CAD build for the part. Positions are in the model's coordinates, mm. A direction names the side the tool comes from. Coordinates: 2 decimals unless noted, no trailing zeros. Order: outer loops, then holes, each group sorted by start corner. A loop starts at its lowest first (then second) coordinate and runs counter-clockwise, first axis right, second up. Notation, with made-up numbers: (30, 23.25) - (84, 23.25) arc R28 ccw to (84, 53.25) - close; hole circle Ø9 at (82, 64). An arc over 180 degrees is marked (long way). Use one line per item in the form item = value.
```python
from build123d import *

# Parameters (mm, degrees)
SKETCH1_R                 = 14
BOSS_EXTRUDE1_DEPTH       = 18.5
CUT_EXTRUDE1_START        = -13.5
SKETCH2_R                 = 14
SKETCH2_R_2               = 5
CUT_EXTRUDE1_DEPTH        = 13.5
SKETCH3_R                 = 4
CUT_EXTRUDE2_DEPTH        = 22.5
CUT_EXTRUDE3_DEPTH        = 3.75
SKETCH8_R                 = 12.271364757
SKETCH8_R_2               = 6.141449245
CUT_EXTRUDE4_DEPTH        = 2.75
CIRPATTERN1_COUNT         = 4
SKETCH11_R                = 1.5
CUT_EXTRUDE5_DEPTH        = 3
SKETCH12_R                = 21.13637798
CUT_EXTRUDE6_DEPTH        = 17
BOSS_EXTRUDE2_START       = -1.5
BOSS_EXTRUDE2_OUTLINE_R   = 1.5
BOSS_EXTRUDE2_OUTLINE_R_2 = 1.517060808
BOSS_EXTRUDE2_OUTLINE_R_3 = 4
BOSS_EXTRUDE2_OUTLINE_R_4 = 1.426709917
BOSS_EXTRUDE2_DEPTH       = 1.5
FILLET1_R                 = 2.5
SKETCH14_R                = 1.5
SKETCH14_R_2              = 5
CUT_EXTRUDE7_DEPTH        = 14.5


# Read off the part's stored shape, not the designer's step: Boss-Extrude2
with BuildPart() as part:
    # Sketch1 → Boss-Extrude1 (new body)
    with BuildSketch(Plane.XY):
        Circle(SKETCH1_R)
    extrude(amount=BOSS_EXTRUDE1_DEPTH)

    # Sketch2 → Cut-Extrude1 (cut)
    with BuildSketch(Plane.XY.offset(18.5).offset(CUT_EXTRUDE1_START)):
        Circle(SKETCH2_R)
        Circle(SKETCH2_R_2, mode=Mode.SUBTRACT)
    extrude(amount=CUT_EXTRUDE1_DEPTH, mode=Mode.SUBTRACT)

    # Sketch3 → Cut-Extrude2 (cut)
    with BuildSketch(Plane.XY.offset(18.5)):
        Circle(SKETCH3_R)
    extrude(amount=-CUT_EXTRUDE2_DEPTH, mode=Mode.SUBTRACT)

    # Sketch6 → Cut-Revolve1 (revolve, cut)
    with BuildSketch(Plane(origin=(0, 0, 0), x_dir=(0, 0, -1), z_dir=(1, 0, 0)), mode=Mode.PRIVATE) as cut_revolve1_sk:
        Polygon((-4.949121361, 14), (3.777639186, 16.199586118), (5.061522468, 10.233304984), align=None)
    revolve(cut_revolve1_sk.sketch.rotate(Axis((0, 0, 19.921792725), (0, 0, -1)), 90), axis=Axis((0, 0, 19.921792725), (0, 0, -1)), mode=Mode.SUBTRACT)

    # Sketch7 → Cut-Extrude3 (cut)
    with BuildSketch(Plane(origin=(0, 0, 0), x_dir=(-1, 0, 0), z_dir=(0, 0, -1))):
        with BuildLine():
            Line((3, 15.639460569), (3, 11.87697352))
            add(Edge.make_bspline(
                [(3, 11.87697352), (3.121054504, 3.206614769), (11.87697352, 3)],
                knots=[0, 0, 0, 1, 1, 1], degree=2))
            Line((11.87697352, 3), (17.86108213, 3))
            Line((17.86108213, 3), (14.869027825, 14.316513241))
            Line((14.869027825, 14.316513241), (3, 15.639460569))
        make_face()
    cut_extrude3 = extrude(amount=-CUT_EXTRUDE3_DEPTH, mode=Mode.SUBTRACT)

    # Sketch8 → Cut-Extrude4 (cut)
    with BuildSketch(Plane.XY.offset(5)):
        Circle(SKETCH8_R)
        Circle(SKETCH8_R_2, mode=Mode.SUBTRACT)
    extrude(amount=-CUT_EXTRUDE4_DEPTH, mode=Mode.SUBTRACT)

    # Sketch9 → Cut-Revolve2 (revolve, cut)
    with BuildSketch(Plane(origin=(0, 0, 0), x_dir=(1, 0, 0), z_dir=(0, 1, 0)), mode=Mode.PRIVATE) as cut_revolve2_sk:
        Polygon((-12.001476603, -2.22152714), (-13.001507243, -5.36905248), (-11.155114973, -5.36905248), align=None)
    revolve(cut_revolve2_sk.sketch.rotate(Axis((0, 0, -1.742471472), (0, 0, 1)), 180), axis=Axis((0, 0, -1.742471472), (0, 0, 1)), mode=Mode.SUBTRACT)

    # Sketch10 → Cut-Revolve3 (revolve, cut)
    with BuildSketch(Plane(origin=(0, 0, 0), x_dir=(1, 0, 0), z_dir=(0, 1, 0)), mode=Mode.PRIVATE) as cut_revolve3_sk:
        Polygon((-5, -5), (-6.141449245, -2.28305418), (-6.572257958, -5.413209842), align=None)
    revolve(cut_revolve3_sk.sketch.rotate(Axis((0, 0, 0), (0, 0, -1)), 180), axis=Axis((0, 0, 0), (0, 0, -1)), mode=Mode.SUBTRACT)

    # CirPattern1: Cut-Extrude3 ×4 about axis
    cirpattern1_axis = Axis((0, 0, 3.75), (0, 0, 1))
    for i in range(1, CIRPATTERN1_COUNT):
        add(cut_extrude3.rotate(cirpattern1_axis, i * 360 / CIRPATTERN1_COUNT), mode=Mode.SUBTRACT)

    # Sketch11 → Cut-Extrude5 (cut)
    with BuildSketch(Plane(origin=(0, 0, 0), x_dir=(-1, 0, 0), z_dir=(0, 0, -1))):
        with Locations((0, 8)):
            Circle(SKETCH11_R)
        with Locations((0, -8)):
            Circle(SKETCH11_R)
        with Locations((-10, 0)):
            Circle(SKETCH11_R)
        with Locations((10, 0)):
            Circle(SKETCH11_R)
    extrude(amount=-CUT_EXTRUDE5_DEPTH, mode=Mode.SUBTRACT)

    # Sketch12 → Cut-Extrude6 (cut)
    with BuildSketch(Plane.XY.offset(18.5)):
        Circle(SKETCH12_R)
    extrude(amount=-CUT_EXTRUDE6_DEPTH, mode=Mode.SUBTRACT)

    # Boss-Extrude2 outline → Boss-Extrude2 (add)
    # profile 1 of 7: a face of its own
    with BuildSketch(Plane(origin=(0, 0, 0), x_dir=(-1, 0, 0), z_dir=(0, 0, -1)).offset(BOSS_EXTRUDE2_START)):
        with BuildLine():
            add(Edge.make_bspline(
                [(3.00190242, 11.760729011), (3.000755095, 11.818659857), (3, 11.87697352)],
                knots=[0.993159083, 0.993159083, 0.993159083, 1, 1, 1], degree=2))
            Line((3, 11.87697352), (3, 19.773719933))
            ThreePointArc((3, 19.773719933), (-0.004378174, 19.999999521), (-3.00865699, 19.772404586))
            Line((-3.00865699, 19.772404586), (-3.008656992, 11.602060374))
            add(Edge.make_bspline(
                [(-5.368896851, 5.233886038), (-3.175302873, 7.384008673), (-3.008656992, 11.602060374)],
                knots=[0.4948048, 0.4948048, 0.4948048, 0.984177857, 0.984177857, 0.984177857], degree=2))
            add(Edge.make_bspline(
                [(-5.368896851, 5.233886038), (-7.55686142, 3.085160323), (-11.760729011, 3.00190242)],
                knots=[0.496734279, 0.496734279, 0.496734279, 0.993159083, 0.993159083, 0.993159083], degree=2))
            add(Edge.make_bspline(
                [(-11.760729011, 3.00190242), (-11.818659857, 3.000755095), (-11.87697352, 3)],
                knots=[0.993159083, 0.993159083, 0.993159083, 1, 1, 1], degree=2))
            Line((-11.87697352, 3), (-19.773719933, 3))
            ThreePointArc((-19.773719933, 3), (-19.999999521, -0.004378174), (-19.772404586, -3.00865699))
            Line((-19.772404586, -3.00865699), (-11.602060374, -3.008656992))
            add(Edge.make_bspline(
                [(-5.233886038, -5.368896851), (-7.384008673, -3.175302873), (-11.602060374, -3.008656992)],
                knots=[0.4948048, 0.4948048, 0.4948048, 0.984177857, 0.984177857, 0.984177857], degree=2))
            add(Edge.make_bspline(
                [(-5.233886038, -5.368896851), (-3.085160323, -7.55686142), (-3.00190242, -11.760729011)],
                knots=[0.496734279, 0.496734279, 0.496734279, 0.993159083, 0.993159083, 0.993159083], degree=2))
            add(Edge.make_bspline(
                [(-3.00190242, -11.760729011), (-3.000755095, -11.818659857), (-3, -11.87697352)],
                knots=[0.993159083, 0.993159083, 0.993159083, 1, 1, 1], degree=2))
            Line((-3, -11.87697352), (-3, -19.773719933))
            ThreePointArc((-3, -19.773719933), (0.004378174, -19.999999521), (3.00865699, -19.772404586))
            Line((3.00865699, -19.772404586), (3.008656992, -11.602060374))
            add(Edge.make_bspline(
                [(5.368896851, -5.233886038), (3.175302873, -7.384008673), (3.008656992, -11.602060374)],
                knots=[0.4948048, 0.4948048, 0.4948048, 0.984177857, 0.984177857, 0.984177857], degree=2))
            add(Edge.make_bspline(
                [(5.368896851, -5.233886038), (7.55686142, -3.085160323), (11.760729011, -3.00190242)],
                knots=[0.496734279, 0.496734279, 0.496734279, 0.993159083, 0.993159083, 0.993159083], degree=2))
            add(Edge.make_bspline(
                [(11.760729011, -3.00190242), (11.818659857, -3.000755095), (11.87697352, -3)],
                knots=[0.993159083, 0.993159083, 0.993159083, 1, 1, 1], degree=2))
            Line((11.87697352, -3), (19.773719933, -3))
            ThreePointArc((19.773719933, -3), (19.999999521, 0.004378174), (19.772404586, 3.00865699))
            Line((19.772404586, 3.00865699), (11.602060374, 3.008656992))
            add(Edge.make_bspline(
                [(5.233886023, 5.368896867), (7.384008658, 3.175302874), (11.602060374, 3.008656992)],
                knots=[0.494804799, 0.494804799, 0.494804799, 0.984177857, 0.984177857, 0.984177857], degree=2))
            add(Edge.make_bspline(
                [(5.233886023, 5.368896867), (3.085160322, 7.556861435), (3.00190242, 11.760729011)],
                knots=[0.496734281, 0.496734281, 0.496734281, 0.993159083, 0.993159083, 0.993159083], degree=2))
        make_face()
        with Locations((0, -8)):
            Circle(BOSS_EXTRUDE2_OUTLINE_R, mode=Mode.SUBTRACT)
        with Locations((-10, 0)):
            Circle(BOSS_EXTRUDE2_OUTLINE_R_2, mode=Mode.SUBTRACT)
        Circle(BOSS_EXTRUDE2_OUTLINE_R_3, mode=Mode.SUBTRACT)
        with Locations((0, 8)):
            Circle(BOSS_EXTRUDE2_OUTLINE_R, mode=Mode.SUBTRACT)
        with Locations((10, 0)):
            Circle(BOSS_EXTRUDE2_OUTLINE_R, mode=Mode.SUBTRACT)
    # profile 2 of 7: a face of its own
    with BuildSketch(Plane(origin=(0, 0, 0), x_dir=(-1, 0, 0), z_dir=(0, 0, -1)).offset(BOSS_EXTRUDE2_START)):
        with BuildLine():
            add(Edge.make_bspline(
                [(11.60206042, 3.00865699), (7.383951275, 3.179568286), (5.233886023, 5.368896867)],
                knots=[0, 0, 0, 0.496734281, 0.496734281, 0.496734281], degree=2))
            add(Edge.make_bspline(
                [(5.233886023, 5.368896867), (7.384008658, 3.175302874), (11.60206042, 3.00865699)],
                knots=[0.494804799, 0.494804799, 0.494804799, 0.984177857, 0.984177857, 0.984177857], degree=2))
        make_face()
    # profile 3 of 7: a face of its own
    with BuildSketch(Plane(origin=(0, 0, 0), x_dir=(-1, 0, 0), z_dir=(0, 0, -1)).offset(BOSS_EXTRUDE2_START)):
        with BuildLine():
            add(Edge.make_bspline(
                [(-5.368896851, 5.233886038), (-3.175302873, 7.384008673), (-3.008656992, 11.602060374)],
                knots=[0.4948048, 0.4948048, 0.4948048, 0.984177857, 0.984177857, 0.984177857], degree=2))
            add(Edge.make_bspline(
                [(-3.008656992, 11.602060374), (-3.179568285, 7.383951289), (-5.368896851, 5.233886038)],
                knots=[0, 0, 0, 0.496734279, 0.496734279, 0.496734279], degree=2))
        make_face()
    # profile 4 of 7: a face of its own
    with BuildSketch(Plane(origin=(0, 0, 0), x_dir=(-1, 0, 0), z_dir=(0, 0, -1)).offset(BOSS_EXTRUDE2_START)):
        with BuildLine():
            add(Edge.make_bspline(
                [(3.00865699, -11.60206042), (3.179568285, -7.383951289), (5.368896851, -5.233886038)],
                knots=[0, 0, 0, 0.496734279, 0.496734279, 0.496734279], degree=2))
            add(Edge.make_bspline(
                [(5.368896851, -5.233886038), (3.175302873, -7.384008673), (3.00865699, -11.60206042)],
                knots=[0.4948048, 0.4948048, 0.4948048, 0.984177857, 0.984177857, 0.984177857], degree=2))
        make_face()
    # profile 5 of 7: a face of its own
    with BuildSketch(Plane(origin=(0, 0, 0), x_dir=(-1, 0, 0), z_dir=(0, 0, -1)).offset(BOSS_EXTRUDE2_START)):
        with BuildLine():
            add(Edge.make_bspline(
                [(-5.233886038, -5.368896851), (-7.384008673, -3.175302873), (-11.602060374, -3.008656992)],
                knots=[0.4948048, 0.4948048, 0.4948048, 0.984177857, 0.984177857, 0.984177857], degree=2))
            add(Edge.make_bspline(
                [(-11.602060374, -3.008656992), (-7.383951289, -3.179568285), (-5.233886038, -5.368896851)],
                knots=[0, 0, 0, 0.496734279, 0.496734279, 0.496734279], degree=2))
        make_face()
    # profile 6 of 7: a face of its own
    with BuildSketch(Plane(origin=(0, 0, 0), x_dir=(-1, 0, 0), z_dir=(0, 0, -1)).offset(BOSS_EXTRUDE2_START)):
        Circle(BOSS_EXTRUDE2_OUTLINE_R_3)
    # profile 7 of 7: a face of its own
    with BuildSketch(Plane(origin=(0, 0, 0), x_dir=(-1, 0, 0), z_dir=(0, 0, -1)).offset(BOSS_EXTRUDE2_START)):
        with Locations((0, 8)):
            Circle(BOSS_EXTRUDE2_OUTLINE_R)
        with Locations((0, 8)):
            Circle(BOSS_EXTRUDE2_OUTLINE_R_4, mode=Mode.SUBTRACT)
    extrude(amount=BOSS_EXTRUDE2_DEPTH)

    # Fillet1
    fillet1_edges = [part.edges().sort_by_distance(p)[0] for p in [
        (-19.772404586, 3.00865699, 0.75),
        (-19.773719933, -3, 0.75),
        (-3.00865699, -19.772404586, 0.75),
        (3, -19.773719933, 0.75),
        (19.772404586, -3.00865699, 0.75),
        (19.773719933, 3, 0.75),
        (-3, 19.773719933, 0.75),
        (3.00865699, 19.772404586, 0.75),
    ]]
    fillet(fillet1_edges, radius=FILLET1_R)

    # Sketch14 → Cut-Extrude7 (cut)
    with BuildSketch(Plane(origin=(0, 0, 0), x_dir=(-1, 0, 0), z_dir=(0, 0, -1))):
        with Locations((0, 17.261717903)):
            Circle(SKETCH14_R)
        with Locations((17.261717903, 0)):
            Circle(SKETCH14_R)
        with Locations((0, -17.261717903)):
            Circle(SKETCH14_R)
        with Locations((-17.261717903, 0)):
            Circle(SKETCH14_R)
        Circle(SKETCH14_R_2)
    extrude(amount=-CUT_EXTRUDE7_DEPTH, mode=Mode.SUBTRACT)


solid = part.part
```
Item 1: Cut at D-D, the plane z = 0.8. State how many separate pieces and enclosed holes the cut face has, plus the area to 3 significant figures.
Derived:
separate_pieces = 1
enclosed_holes = 9
area = 355 mm²
Item 2: Two-plate mould, pull along Y, no slides. Class faces 1 (the face through (-5, -3, 1.5)), 2 (the face through (-19.22, -2.31, 0.74)), 3 (the face through (-0.806, 18.527, 0.74)): +Y half, -Y half, draft (parallel to the pull), parting line (faces both ways), or undercut.
Derived:
face_1 = draft
face_2 = -Y half
face_3 = undercut
Item 3: Drop flat-ended pins along their axis: pin 1 (8 mm diameter, centred on x = 0, y = 0, fed in from -Z); pin 2 (3.5 mm diameter, centred on x = 0, y = 17.26, fed in from -Z); pin 3 (0.8 mm diameter, centred on y = -14.5, z = 1, fed in from +X). Give the stop position or say it passes through.
Derived:
pin_1 = through
pin_2 = 0
pin_3 = 3
Item 4: Cut at A-A, the plane x = 0. Write the cut outline in (y, z), plus the area to 3 significant figures.
Derived:
outline = (-20, 0) - (-18.76, 0) - (-18.76, 1.5) - (-20, 1.5) - close; (-15.76, 0) - (-9.5, 0) - (-9.5, 1.5) - (-15.76, 1.5) - close; (-6.5, 0) - (-5, 0) - (-5, 1.5) - (-6.5, 1.5) - close; (5, 0) - (6.57, 0) - (6.57, 1.5) - (5, 1.5) - close; (9.43, 0) - (15.76, 0) - (15.76, 1.5) - (9.43, 1.5) - close; (18.76, 0) - (20, 0) - (20, 1.5) - (18.76, 1.5) - close
area = 27.2 mm²
Item 5: Drill centre lines: line 1 (Y direction, x = 0, z = 0.35); line 2 (X direction, y = 2.5, z = 0.5); line 3 (Y direction, x = -14, z = 0.6). Where is each one in solid material? Low to high. Write a range as [from, to].
Derived:
line_1 = [-20, -18.76], [-15.76, -9.5], [-6.5, -5], [5, 6.57], [9.43, 15.76], [18.76, 20]
line_2 = [-19, -4.33], [4.33, 18.99]
line_3 = [-3, 3.01]
Item 6: Cut at C-C, the plane y = -14.5. Write the cut outline in (x, z), plus the area to 3 significant figures.
Derived:
outline = (-3.01, 0) - (3, 0) - (3, 1.5) - (-3.01, 1.5) - close
area = 9.01 mm²
Item 7: 3-axis set-ups, long thin cutter, end or side, ignore diameter. For faces 4 (the face through (-15, -3, 1)), 5 (the face through (15, 3, 1)), 6 (the face through (15, -3.009, 1)): which of +Z, -Z, +X, -X, +Y, -Y reach the whole face in a straight line?
Derived:
face_4 = +Z, -Z, -X, -Y
face_5 = +Z, -Z, +X, +Y
face_6 = +Z, -Z, +X, -Y
Item 8: Cut at B-B, the plane y = 0. Write the cut outline in (x, z).
Derived:
outline = (-20, 0) - (-18.76, 0) - (-18.76, 1.5) - (-20, 1.5) - close; (-15.76, 0) - (-11.5, 0) - (-11.5, 1.5) - (-15.76, 1.5) - close; (-8.5, 0) - (-5, 0) - (-5, 1.5) - (-8.5, 1.5) - close; (5, 0) - (8.5, 0) - (8.5, 1.5) - (5, 1.5) - close; (11.5, 0) - (15.76, 0) - (15.76, 1.5) - (11.5, 1.5) - close; (18.76, 0) - (20, 0) - (20, 1.5) - (18.76, 1.5) - close
